```python
from build123d import *

# Parameters (mm, degrees)
SKETCH4_R           = 2
BOSS_EXTRUDE1_DEPTH = 5.95
SKETCH5_R           = 1.5
CUT_EXTRUDE1_DEPTH  = 5
SKETCH6_R           = 1.5
CUT_EXTRUDE2_DEPTH  = 5
SKETCH7_R           = 4.25
BOSS_EXTRUDE2_DEPTH = 4.3
SKETCH8_R           = 2.8
CUT_EXTRUDE3_DEPTH  = 0.1
CUT_EXTRUDE4_DEPTH  = 1.5
SKETCH10_R          = 6.5
SKETCH10_R_2        = 5.5
CUT_EXTRUDE5_DEPTH  = 0.1


with BuildPart() as part:
    # Sketch3 → Revolve1 (revolve)
    with BuildSketch(Plane(origin=(0, 0, 0), x_dir=(0, 0, -1), z_dir=(1, 0, 0)), mode=Mode.PRIVATE) as revolve1_sk:
        Polygon((-29.5, 0), (-29.5, 14), (-25.5, 28.93), (-8.5, 28.93), (-8.5, 26.93), (-8, 26.93), (-8, 28.93), (-5, 28.93), (0, 17.75), (0, 9), (-1.5, 7.5), (-1.5, 0), align=None)
    revolve(revolve1_sk.sketch.rotate(Axis((0, 0, 66.283384922), (0, 0, -1)), 90), axis=Axis((0, 0, 66.283384922), (0, 0, -1)))

    # Sketch4 → Boss-Extrude1 (add)
    with BuildSketch(Plane.XY.offset(29.5)):
        with Locations(Location((0, 0, 0), (0, 0, 180))):
            Circle(SKETCH4_R)
    extrude(amount=BOSS_EXTRUDE1_DEPTH)

    # Sketch5 → Cut-Extrude1 (cut)
    with BuildSketch(Plane.XY.offset(29.5)):
        with Locations((0, 6)):
            Circle(SKETCH5_R)
        with Locations((6, 0)):
            Circle(SKETCH5_R)
        with Locations((0, -6)):
            Circle(SKETCH5_R)
        with Locations((-6, 0)):
            Circle(SKETCH5_R)
    extrude(amount=-CUT_EXTRUDE1_DEPTH, mode=Mode.SUBTRACT)

    # Sketch6 → Cut-Extrude2 (cut)
    with BuildSketch(Plane(origin=(0, 0, 0), x_dir=(-1, 0, 0), z_dir=(0, 0, -1))):
        with Locations((0, 12.5)):
            Circle(SKETCH6_R)
        with Locations((12.5, 0)):
            Circle(SKETCH6_R)
        with Locations((0, -12.5)):
            Circle(SKETCH6_R)
        with Locations((-12.5, 0)):
            Circle(SKETCH6_R)
    extrude(amount=-CUT_EXTRUDE2_DEPTH, mode=Mode.SUBTRACT)

    # Sketch7 → Boss-Extrude2 (add)
    with BuildSketch(Plane(origin=(0, 0, 1.5), x_dir=(-1, 0, 0), z_dir=(0, 0, -1))):
        with Locations(Location((0, 0, 0), (0, 0, 180))):
            Circle(SKETCH7_R)
    extrude(amount=BOSS_EXTRUDE2_DEPTH)

    # Sketch8 → Cut-Extrude3 (cut)
    with BuildSketch(Plane(origin=(0, 0, -2.8), x_dir=(-1, 0, 0), z_dir=(0, 0, -1))):
        Circle(SKETCH8_R)
    extrude(amount=-CUT_EXTRUDE3_DEPTH, mode=Mode.SUBTRACT)

    # Sketch9 → Cut-Extrude4 (cut)
    with BuildSketch(Plane(origin=(0, 0, -2.7), x_dir=(-1, 0, 0), z_dir=(0, 0, -1))):
        Polygon((0, -1.154700538), (1, -0.577350269), (1, 0.577350269), (0, 1.154700538), (-1, 0.577350269), (-1, -0.577350269), align=None)
    extrude(amount=-CUT_EXTRUDE4_DEPTH, mode=Mode.SUBTRACT)

    # Sketch10 → Cut-Extrude5 (cut)
    with BuildSketch(Plane(origin=(0, 0, 1.5), x_dir=(-1, 0, 0), z_dir=(0, 0, -1))):
        Circle(SKETCH10_R)
        Circle(SKETCH10_R_2, mode=Mode.SUBTRACT)
    extrude(amount=-CUT_EXTRUDE5_DEPTH, mode=Mode.SUBTRACT)


solid = part.part
```
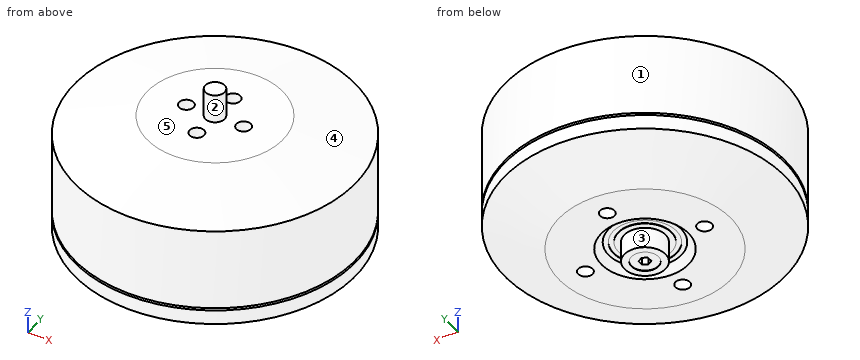
CAD build for the part. Positions are in the model's coordinates, mm. Face numbers are marked on the shaded views. A direction names the side the tool comes from. Coordinates: 2 decimals unless noted, no trailing zeros. Order: outer loops, then holes, each group sorted by start corner. A loop starts at its lowest first (then second) coordinate and runs counter-clockwise, first axis right, second up. Notation, with made-up numbers: M 44,22 L 67,22 A23 ccw 67,53 Z; hole C 80.25,18.25 d1. An arc over 180 degrees is marked long. Write each question's results on one line, items separated by ' | '. Start each with the question number.
Q1. Flat gauge pins, fed straight in: P1, Ø3.5, axis at x = 0, y = -6.5, coming from the +Z side; P2, Ø3.5, axis at x = 12.5, y = 0, coming from the -Z side; P3, Ø3, axis at x = 15, z = 14.5, coming from the -Y side. Where does each tip first touch, or does it go through?
Q2. Pull direction Y, two halves, no side cores. Call the marked faces 3, 4 and 5: +Y half, -Y half, draft (parallel to the pull), parting line (faces both ways), or undercut.
Q3. Drill centre lines: probe 1 along Z at (x, y) = (11.5, -3); probe 2 along Z at (x, y) = (6, -1); probe 3 along Z at (x, y) = (16.5, -22.5). Where is each one in solid material? Low to high. Write a range as from..to.
Q4. Which spindle directions (+Z, -Z, +X, -X, +Y, -Y) get a long thin tool onto all of the face, cutting with end or side? Do the marked faces 1 and 2. Say none if no direction does.
Q5. Cut at A-A (z = 22). List the corners of the cut face in (x, y).
Found:
1) P1: z = 29.5 | P2: z = 0 | P3: y = -25.59
2) face 3: undercut | face 4: parting line | face 5: draft
3) probe 1: 0..29.5 | probe 2: 1.6..24.5 | probe 3: 4.54..8, 8.5..25.78
4) face 1: +Z, -Z | face 2: +Z
5) outline: C 0,0 d57.86
